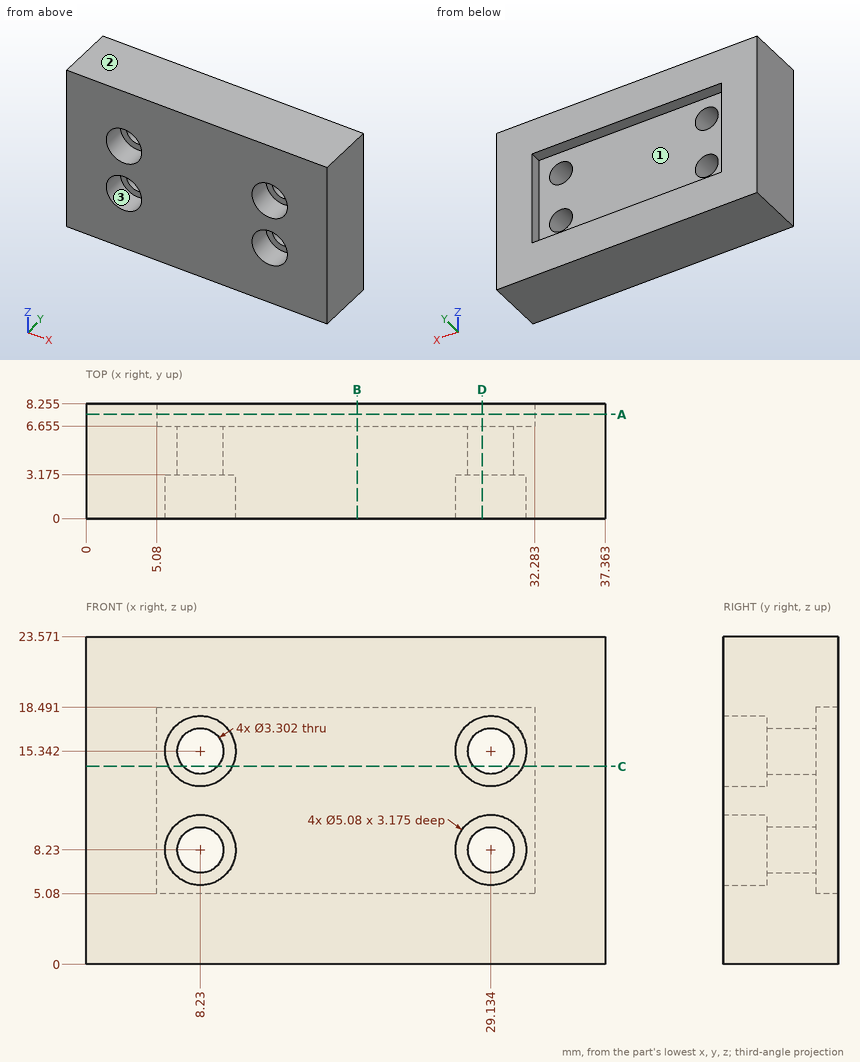
Input: dimensioned drawing with shaded views. Units: mm. Origin: part minimum x, y, z. A direction names the side the tool comes from. Give positions to 0.01 mm unless a question says otherwise; leave off trailing zeros. Order: outer loops, then holes, each group sorted by start corner. A loop starts at its lowest first (then second) coordinate and runs counter-clockwise, first axis right, second up. Notation, with made-up numbers: (17.25, 27.25) -> (33.25, 27.25) arc R17 ccw to (33.25, 45.25) -> close; hole circle Ø2 at (86.5, 18). An arc over 180 degrees is marked (long way). Answer as a JSON object with one key per item and string values.
Q1. Section A-A (y = 7.5). Output: boundary loops of the cut face in (x, z).
Entries:
{"outline": "(0, 0) -> (37.36, 0) -> (37.36, 23.57) -> (0, 23.57) -> close; hole (5.08, 5.08) -> (32.28, 5.08) -> (32.28, 18.49) -> (5.08, 18.49) -> close"}
Q2. First-contact query: pin 1 (10.5 mm diameter, centred on x = 23.5, z = 12.5, fed in from +Y) (1 decimal); pin 2 (2.5 mm diameter, centred on x = 30, z = 16, fed in from -Y) (3 decimals). Flat tips, straight axial feed; report the tip coordinate or a pass-through.
Entries:
{"pin 1": "stops at y = 6.7", "pin 2": "stops at y = 3.175"}
Q3. Section B-B (x = 19.5). Output: boundary loops of the cut face in (y, z) (1 decimal), plus the area to 3 significant figures.
Entries:
{"outline": "(0, 0) -> (8.3, 0) -> (8.3, 5.1) -> (6.7, 5.1) -> (6.7, 18.5) -> (8.3, 18.5) -> (8.3, 23.6) -> (0, 23.6) -> close", "area": "173 mm^2"}
Q4. Material intervals for probe 1 along X at (y, z) = (7.5, 10.5); probe 2 along X at (y, z) = (1.5, 14.5) (1 decimal); probe 3 along Z at (x, y) = (8.5, 4.5), sorted ascending.
Entries:
{"probe 1": "x = 0 to 5.08, 32.28 to 37.36", "probe 2": "x = 0 to 5.8, 10.6 to 26.7, 31.5 to 37.4", "probe 3": "z = 0 to 6.6, 9.86 to 13.71, 16.97 to 23.57"}
Q5. Section D-D (x = 28.5). Output: boundary loops of the cut face in (y, z) (1 decimal), plus the area to 3 significant figures.
Entries:
{"outline": "(0, 0) -> (8.3, 0) -> (8.3, 5.1) -> (6.7, 5.1) -> (6.7, 6.7) -> (3.2, 6.7) -> (3.2, 5.8) -> (0, 5.8) -> close; (0, 10.7) -> (3.2, 10.7) -> (3.2, 9.8) -> (6.7, 9.8) -> (6.7, 13.8) -> (3.2, 13.8) -> (3.2, 12.9) -> (0, 12.9) -> close; (0, 17.8) -> (3.2, 17.8) -> (3.2, 16.9) -> (6.7, 16.9) -> (6.7, 18.5) -> (8.3, 18.5) -> (8.3, 23.6) -> (0, 23.6) -> close", "area": "121 mm^2"}
Q6. Section C-C (z = 14.25). Output: boundary loops of the cut face in (x, y) (1 decimal).
Entries:
{"outline": "(0, 0) -> (5.9, 0) -> (5.9, 3.2) -> (7, 3.2) -> (7, 6.7) -> (5.1, 6.7) -> (5.1, 8.3) -> (0, 8.3) -> close; (9.5, 3.2) -> (10.5, 3.2) -> (10.5, 0) -> (26.8, 0) -> (26.8, 3.2) -> (27.9, 3.2) -> (27.9, 6.7) -> (9.5, 6.7) -> close; (30.4, 3.2) -> (31.4, 3.2) -> (31.4, 0) -> (37.4, 0) -> (37.4, 8.3) -> (32.3, 8.3) -> (32.3, 6.7) -> (30.4, 6.7) -> close"}
Q7. Access query for the marked faces 1, 2 and 3. Directions: +Z, -Z, +X, -X, +Y, -Y. A direction counts if a zero-diameter tool reaches every point of the face in a straight line with its end or side. Return the directions, or none.
Entries:
{"face 1": "+Y", "face 2": "+Z, +X, -X, +Y, -Y", "face 3": "-Y"}
